Could you check a few things on this model? Use its own coordinates, in mm. Give positions to 0.01 mm unless a question says otherwise; leave off trailing zeros. Order: outer loops, then holes, each group sorted by start corner. A loop starts at its lowest first (then second) coordinate and runs counter-clockwise, first axis right, second up. Notation, with made-up numbers: (67, 45) -> (103, 45) arc R30 cw to (103, 72) -> close; hole circle Ø9 at (-33.75, 17.5). An arc over 180 degrees is marked (long way). Write each question's results on one line, items separated by ' | '.
Autodesk Inventor part; units mm, degrees
ref_plane "YZ Plane" through (0, 0, 0) normal (1, 0, 0) x (0, 1, 0)
ref_plane "XZ Plane" through (0, 0, 0) normal (0, 1, 0) x (-1, 0, 0)
ref_plane "XY Plane" through (0, 0, 0) normal (0, 0, 1) x (1, 0, 0)
sketch "Sketch1" plane through (0, 0, 0) normal (0, 1, 0) x (-1, 0, 0)
  line L0 (-50, 195) -> (-50, -195)
  line L1 (50, -195) -> (50, 195)
  circle A0 centre (0, 0) radius 40
  line L2 (70, 37.125) -> (-67, 37.125) construction
  line L3 (70, -37.125) -> (-81, -37.125) construction
  circle A1 centre (37.125, 37.125) radius 3.25
  circle A2 centre (37.125, -37.125) radius 3.25
  circle A3 centre (-37.125, -37.125) radius 3.25
  circle A4 centre (-37.125, 37.125) radius 3.25
  line L4 (50, 195) -> (-50, 195)
  line L5 (50, -195) -> (-50, -195)
  line L6 (97, 172.5) -> (-97, 172.5) construction
  line L7 (88, -172.5) -> (-85, -172.5) construction
  line L8 (-25, 119) -> (-25, -106) construction
  line L9 (25, -106) -> (25, 119) construction
  circle A5 centre (25, 172.5) radius 4.25
  circle A6 centre (-25, 172.5) radius 4.25
  circle A7 centre (-25, -172.5) radius 4.25
  circle A8 centre (25, -172.5) radius 4.25
  dimension "d0" = 80
  dimension "d5" = 74.25
  dimension "d6" = 37.125
  dimension "d7" = 6.5
  dimension "d12" = 74.25
  dimension "d14" = 37.125
  dimension "d15" = 37.125
  dimension "d16" = 37.125
  dimension "d24" = 50
  dimension "d25" = 25
  dimension "d26" = 8.5
  dimension "d29" = 390
  dimension "d30" = 195
  dimension "d31" = 100
  dimension "d32" = 50
  dimension "d33" = 22.5
  dimension "d34" = 22.5
extrude "Extrusion2" add sketch "Sketch1" along normal blind 10
properties part number "1223_Motor Plate_V1" material "Wood (Birch)"
Q1. Thinking about a two-plate mould opening in X: for faces 1 (the flat face through (-50, 5, -3)), 2 (the flat face through (-1, 5, 195)), 3 (the cylindrical face through (-24.447, 4.93, 168.286)), which applies, +X half, -X half, draft (parallel to the pull), parting line (faces both ways), or undercut?
Here are the results:
face 1: -X half | face 2: draft | face 3: undercut
Q2. I need wall thicknesses on line 1 along X through (y, z) = (0.5, -173); line 2 along Z through (x, y) = (-25, 6.75); line 3 along Z through (x, y) = (27, 7.75). Which ranges of each line are inside material? Lowest first, please.
Here are the results:
line 1: x = -50 to -29.22, -20.78 to 20.78, 29.22 to 50 | line 2: z = -195 to -176.75, -168.25 to -31.22, 31.22 to 168.25, 176.75 to 195 | line 3: z = -195 to -176.25, -168.75 to -29.51, 29.51 to 168.75, 176.25 to 195
Q3. Suppose I cut it at B-B on z = 0. Please give me the cut outline in (x, y), and give its area (3 significant figures).
Here are the results:
outline: (-50, 0) -> (-40, 0) -> (-40, 10) -> (-50, 10) -> close; (40, 0) -> (50, 0) -> (50, 10) -> (40, 10) -> close | area: 200 mm²
Q4. Suppose I cut it at D-D on x = -25. Please give me the cut outline in (y, z).
Here are the results:
outline: (0, -195) -> (10, -195) -> (10, -176.75) -> (0, -176.75) -> close; (0, -168.25) -> (10, -168.25) -> (10, -31.22) -> (0, -31.22) -> close; (0, 31.22) -> (10, 31.22) -> (10, 168.25) -> (0, 168.25) -> close; (0, 176.75) -> (10, 176.75) -> (10, 195) -> (0, 195) -> close
Q5. I'm going to push a flat-ended pin straight in: pin 1 Ø6 at (x, z) = (37.125, 37.125) entering from +Y. Where does the tip first touch, or does it pass through?
Here are the results:
pin 1: passes through
Q6. Suppose I cut it at C-C on y = 2. State how many separate pieces and enclosed holes the cut face has, and give its area (3 significant figures).
Here are the results:
separate pieces: 1 | enclosed holes: 9 | area: 33,600 mm²
Q7. Suppose I cut it at A-A on x = -1. Please give me the cut outline in (y, z), and give its area (3 significant figures).
Here are the results:
outline: (0, -195) -> (10, -195) -> (10, -39.99) -> (0, -39.99) -> close; (0, 39.99) -> (10, 39.99) -> (10, 195) -> (0, 195) -> close | area: 3,100 mm²
